Work out the finished part from the listing and answer in its coordinate system (mm). Give positions to 0.01 mm unless a question says otherwise; leave off trailing zeros. Order: outer loops, then holes, each group sorted by start corner. A loop starts at its lowest first (then second) coordinate and runs counter-clockwise, first axis right, second up. Notation, with made-up numbers: M 43.25,68 L 88.25,68 A20 cw 88.25,77 Z; hole C -16.75,25.5 d3. An arc over 180 degrees is marked long. One line per item, written item: value.
from build123d import *

# Parameters (mm, degrees)
SKETCH1_W           = 254
SKETCH1_H           = 101.6
SKETCH1_R           = 1.905
SKETCH1_R_2         = 1.651
SKETCH1_W_2         = 31.242
SKETCH1_H_2         = 14.732
BOSS_EXTRUDE1_DEPTH = 4


with BuildPart() as part:
    # Sketch1 → Boss-Extrude1 (new body)
    with BuildSketch(Plane.XY):
        with Locations((127, 50.8)):
            Rectangle(SKETCH1_W, SKETCH1_H)
        with Locations((34.036, 24.765)):
            Circle(SKETCH1_R, mode=Mode.SUBTRACT)
        with Locations((92.964, 24.765)):
            Circle(SKETCH1_R, mode=Mode.SUBTRACT)
        with Locations((161.036, 24.765)):
            Circle(SKETCH1_R, mode=Mode.SUBTRACT)
        with Locations((219.964, 24.765)):
            Circle(SKETCH1_R, mode=Mode.SUBTRACT)
        with Locations((33.02, 78.74)):
            Circle(SKETCH1_R_2, mode=Mode.SUBTRACT)
        with Locations((33.02, 96.52)):
            Circle(SKETCH1_R_2, mode=Mode.SUBTRACT)
        with Locations((220.98, 78.74)):
            Circle(SKETCH1_R_2, mode=Mode.SUBTRACT)
        with Locations((220.98, 96.52)):
            Circle(SKETCH1_R_2, mode=Mode.SUBTRACT)
        with Locations((15.24, 11.684)):
            Circle(SKETCH1_R_2, mode=Mode.SUBTRACT)
        with Locations((15.24, 29.464)):
            Circle(SKETCH1_R_2, mode=Mode.SUBTRACT)
        with Locations((238.76, 29.464)):
            Circle(SKETCH1_R_2, mode=Mode.SUBTRACT)
        with Locations((238.76, 11.684)):
            Circle(SKETCH1_R_2, mode=Mode.SUBTRACT)
        Polygon((63.5, 14.986), (90.551, 14.986), (90.551, 36.576), (36.449, 36.576), (36.449, 14.986), align=None, mode=Mode.SUBTRACT)
        Polygon((190.5, 14.98050389), (217.992332172, 14.98050389), (217.992332172, 36.57050389), (163.890331935, 36.57050389), (163.890331935, 14.98050389), align=None, mode=Mode.SUBTRACT)
        with Locations((63.5, 55.626)):
            Rectangle(SKETCH1_W_2, SKETCH1_H_2, mode=Mode.SUBTRACT)
        with Locations((190.941332053, 55.626)):
            Rectangle(SKETCH1_W_2, SKETCH1_H_2, mode=Mode.SUBTRACT)
    extrude(amount=BOSS_EXTRUDE1_DEPTH)


solid = part.part
(1) Section A-A, the plane x = 58 is taken. Give the vertices of the cut face in (y, z), then the cut area to 3 significant figures.
Findings:
outline: M 0,0 L 14.99,0 L 14.99,4 L 0,4 Z; M 36.58,0 L 48.26,0 L 48.26,4 L 36.58,4 Z; M 62.99,0 L 101.6,0 L 101.6,4 L 62.99,4 Z
area: 261 mm^2
(2) Find the intervals of material crossed by probe 1 along X at (y, z) = (52.5, 0.35); probe 2 along Y at (x, z) = (195.5, 1.25); probe 3 along X at (y, z) = (32, 3.05), in increasing order. Write a range as from..to.
Findings:
probe 1: x = 0..47.88, 79.12..175.32, 206.56..254
probe 2: y = 0..14.98, 36.57..48.26, 62.99..101.6
probe 3: x = 0..36.45, 90.55..163.89, 217.99..254
(3) Section B-B, the plane z = 3.15 is taken. Give the number of separate pieces and of enclosed holes in the cut face, then the cut area to 3 significant figures.
Findings:
separate pieces: 1
enclosed holes: 16
area: 22,400 mm^2
(4) Given P1, Ø5.5, axis at x = 220.98, y = 96.52, coming from the +Z side; P2, Ø8, axis at x = 200, y = 22.5, coming from the +Z side, each flat-ended and moving along its own axis, determine where each tip first touches the part or whether it passes through.
Findings:
P1: stops at z = 4
P2: passes through
